Could you check a few things on this model? Use its own coordinates, in mm. A direction names the side the tool comes from. Give positions to 0.01 mm unless a question says otherwise; leave off trailing zeros. Order: outer loops, then holes, each group sorted by start corner. A loop starts at its lowest first (then second) coordinate and runs counter-clockwise, first axis right, second up. Notation, with made-up numbers: M 60.25,-8.5 L 66.25,-8.5 A9 cw 66.25,6.5 Z; hole C 33.25,-7 d11. An arc over 180 degrees is marked long. Use a Markdown table: item, result. Add a question column.
Item 1: Suppose I cut it at A-A on x = 2.5. Write out the boundary of the cut face in (y, z).
Item 2: Suppose I cut it at C-C on z = 0.65. Write out the boundary of the cut face in (x, y), plus the area to 3 significant figures.
Item 3: If I drill on L1, parallel to Y at x = 0, z = 2.4; L2, parallel to X at y = 0.75, z = 0.3; L3, parallel to X at y = -1, z = 0.3, over which ranges is the centre line in solid material (lowest first)? Write a range as from..to.
Item 4: For faces 1 (the face through (2, 0, 3)), 2 (the face through (-0.569, 0, 0.5)), 3 (the face through (0, -2.5, 2)), which set-ups out of +Z, -Z, +X, -X, +Y, -Y let a thin tool reach every point of the face, with its end or its side?
Item 5: Suppose I cut it at D-D on y = -1. Write out the boundary of the cut face in (x, z).
Item 6: Suppose I cut it at B-B on z = 1.45. Write out the boundary of the cut face in (x, y), plus the area to 3 significant figures.
Item 7: If we mould it in two halves opening along Y, with no side actions, what happens to faces 4 (the face through (-3, 0, 2)), 5 (the face through (0, -3, 3)), 6 (the face through (0, -3.25, 1))? For each: released by +Y, released by -Y, zero draft, split by the parting line, or undercut.
Item 8: I'm going to push flat-ended pins straight in: pin 1 Ø0.5 at (y, z) = (0, 0.5) entering from +X; pin 2 Ø1.1 at (y, z) = (-0.5, 0.5) entering from -X. Where does each tip first touch, or does it pass through?
from build123d import *

# Parameters (mm, degrees)
SKETCH_1_W          = 7.5
SKETCH_1_H          = 6.5
EXTRUDE_1_DEPTH     = 3
SKETCH_2_W          = 6
SKETCH_2_H          = 5
CUT_EXTRUDE_1_DEPTH = 2
SKETCH_3_R          = 2.25
EXTRUDE_2_DEPTH     = 1
SKETCH_4_R          = 1.5
CUT_EXTRUDE_2_DEPTH = 1
CUT_EXTRUDE_5_DEPTH = 1
SKETCH_9_W          = 0.3
SKETCH_9_H          = 0.8
EXTRUDE_5_DEPTH     = 1.2
SKETCH_11_W         = 0.3
SKETCH_11_H         = 0.8
EXTRUDE_6_DEPTH     = 1.2
FILLET_4_R          = 0.2
FILLET_5_R          = 0.2


with BuildPart() as part:
    # 草图1 → 凸台-拉伸1 (new body)
    with BuildSketch(Plane.XY):
        Rectangle(SKETCH_1_W, SKETCH_1_H)
    extrude(amount=EXTRUDE_1_DEPTH)

    # 草图2 → 切除-拉伸1 (cut)
    with BuildSketch(Plane.XY.offset(3)):
        Rectangle(SKETCH_2_W, SKETCH_2_H)
    extrude(amount=-CUT_EXTRUDE_1_DEPTH, mode=Mode.SUBTRACT)

    # 草图3 → 凸台-拉伸2 (add, symmetric)
    with BuildSketch(Plane.XY.offset(2)):
        with Locations(Location((0, 0, 0), (0, 0, 180))):
            Circle(SKETCH_3_R)
    extrude(amount=EXTRUDE_2_DEPTH, both=True)

    # 草图4 → 切除-拉伸2 (cut, symmetric)
    with BuildSketch(Plane.XY.offset(2)):
        Circle(SKETCH_4_R)
    extrude(amount=CUT_EXTRUDE_2_DEPTH, both=True, mode=Mode.SUBTRACT)

    # 草图8 → 切除-拉伸5 (cut)
    with BuildSketch(Plane(origin=(0, 0, 0), x_dir=(-1, 0, 0), z_dir=(0, 0, -1))):
        with BuildLine():
            Line((-0.56924828, -2.945497648), (-0.56924828, 2.945497648))
            ThreePointArc((-0.56924828, 2.945497648), (-3, 0), (-0.56924828, -2.945497648))
        make_face()
        with BuildLine():
            Line((0.56924828, -2.945497648), (0.56924828, 2.945497648))
            ThreePointArc((0.56924828, 2.945497648), (3, 0), (0.56924828, -2.945497648))
        make_face()
    extrude(amount=-CUT_EXTRUDE_5_DEPTH, mode=Mode.SUBTRACT)

    # 草图9 → 凸台-拉伸5 (add)
    with BuildSketch(Plane(origin=(3.75, 0, 0), x_dir=(0, 0, -1), z_dir=(1, 0, 0))):
        with Locations((-2.85, 2.48)):
            Rectangle(SKETCH_9_W, SKETCH_9_H)
        with Locations((-2.85, -2.48)):
            Rectangle(SKETCH_9_W, SKETCH_9_H)
        with Locations((-2.85, 0)):
            Rectangle(SKETCH_9_W, SKETCH_9_H)
    extrude(amount=EXTRUDE_5_DEPTH)

    # 草图11 → 凸台-拉伸6 (add)
    with BuildSketch(Plane.ZY.offset(3.75)):
        with Locations((2.85, 2.48)):
            Rectangle(SKETCH_11_W, SKETCH_11_H)
        with Locations((2.85, -2.48)):
            Rectangle(SKETCH_11_W, SKETCH_11_H)
        with Locations((2.85, 0)):
            Rectangle(SKETCH_11_W, SKETCH_11_H)
    extrude(amount=EXTRUDE_6_DEPTH)

    # 圆角4
    fillet_4_edges = [part.edges().sort_by_distance(p)[0] for p in [
        (3.75, -0.4, 2.85),
        (3.75, 0, 2.7),
        (4.35, -0.4, 2.7),
        (3.75, 0.4, 2.85),
        (4.35, 0.4, 2.7),
        (4.95, 0, 2.7),
        (-3.75, 2.88, 2.85),
        (-3.75, 2.48, 2.7),
        (-4.35, 2.88, 2.7),
        (-3.75, 2.08, 2.85),
        (-4.35, 2.08, 2.7),
        (-4.95, 2.48, 2.7),
        (-3.75, -2.08, 2.85),
        (-3.75, -2.48, 2.7),
        (-4.35, -2.08, 2.7),
        (-3.75, -2.88, 2.85),
        (-4.35, -2.88, 2.7),
        (-4.95, -2.48, 2.7),
        (-3.75, 0.4, 2.85),
        (-3.75, 0, 2.7),
        (-4.35, 0.4, 2.7),
        (-3.75, -0.4, 2.85),
        (-4.35, -0.4, 2.7),
        (-4.95, 0, 2.7),
        (3.75, 2.08, 2.85),
        (3.75, 2.48, 2.7),
        (4.35, 2.08, 2.7),
        (3.75, 2.88, 2.85),
        (4.35, 2.88, 2.7),
        (4.95, 2.48, 2.7),
        (3.75, -2.88, 2.85),
        (3.75, -2.48, 2.7),
        (4.35, -2.88, 2.7),
        (3.75, -2.08, 2.85),
        (4.35, -2.08, 2.7),
        (4.95, -2.48, 2.7),
    ]]
    fillet(fillet_4_edges, radius=FILLET_4_R)

    # 圆角5
    fillet_5_edges = [part.edges().sort_by_distance(p)[0] for p in [
        (-3.75, 0, 0),
        (3.75, 0, 0),
    ]]
    fillet(fillet_5_edges, radius=FILLET_5_R)


solid = part.part
Findings below:
| question | item | result |
|---|---|---|
| 1 | outline | M -3.25,0 L -1.66,0 L -1.66,1 L -2.5,1 L -2.5,3 L -3.25,3 Z; M 1.66,0 L 3.25,0 L 3.25,3 L 2.5,3 L 2.5,1 L 1.66,1 Z |
| 2 | outline | M -3.75,-3.25 L 3.75,-3.25 L 3.75,3.25 L -3.75,3.25 Z; hole M -0.57,-2.95 L -0.57,2.95 A3 ccw Z; hole M 0.57,-2.95 A3 ccw 0.57,2.95 Z |
| 2 | area | 27.3 mm^2 |
| 3 | L1 | y = -3.25..-2.5, -2.25..-1.5, 1.5..2.25, 2.5..3.25 |
| 3 | L2 | x = -3.75..-2.9, -0.57..0.57, 2.9..3.75 |
| 3 | L3 | x = -3.75..-2.83, -0.57..0.57, 2.83..3.75 |
| 4 | face 1 | +Z, +X, -X, +Y, -Y |
| 4 | face 2 | -Z |
| 4 | face 3 | +Z |
| 5 | outline | M -3.75,0.2 A0.2 ccw -3.55,0 L -2.83,0 L -2.83,1 L -3,1 L -3,3 L -3.75,3 Z; M -2.02,1 L -1.12,1 L -1.12,3 L -2.02,3 Z; M -0.57,0 L 0.57,0 L 0.57,1 L -0.57,1 Z; M 1.12,1 L 2.02,1 L 2.02,3 L 1.12,3 Z; M 2.83,0 L 3.55,0 A0.2 ccw 3.75,0.2 L 3.75,3 L 3,3 L 3,1 L 2.83,1 Z |
| 6 | outline | M -3.75,-3.25 L 3.75,-3.25 L 3.75,3.25 L -3.75,3.25 Z; C 0,0 d4.5; hole M -3,-2.5 L 3,-2.5 L 3,2.5 L -3,2.5 Z; hole C 0,0 d3 |
| 6 | area | 27.6 mm^2 |
| 7 | face 4 | undercut |
| 7 | face 5 | zero draft |
| 7 | face 6 | released by -Y |
| 8 | pin 1 | stops at x = 3.75 |
| 8 | pin 2 | stops at x = -3.75 |
